Could you check a few things on this model? Use its own coordinates, in mm. Give positions to 0.01 mm unless a question says otherwise; leave off trailing zeros. Order: outer loops, then holes, each group sorted by start corner. A loop starts at its lowest first (then second) coordinate and runs counter-clockwise, first axis right, second up.
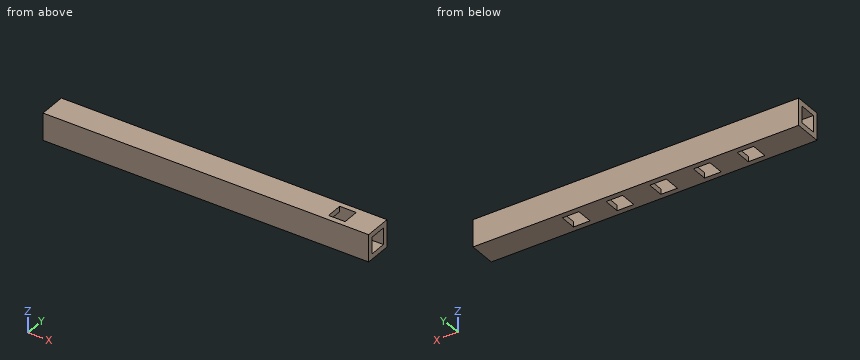
from build123d import *

# Parameters (mm, degrees)
F0_W      = 25.4
F0_H      = 25.4
F1_DEPTH  = 152.4
F1_FACE_W = 25.4
F1_FACE_H = 25.4
F2_DEPTH  = 152.4
F3_W      = 15.494
F3_H      = 15.494
F4_DEPTH  = 304.801
F5_W      = 15.494
F5_H      = 15.494
F6_DEPTH  = 19.05
F7_W      = 15.494
F7_H      = 15.494
F8_DEPTH  = 17.78
F9_DEPTH  = 15.24
F10_DEPTH = 15.24
F11_DEPTH = 15.24
F13_DEPTH = 15.24


with BuildPart() as f1:
    # F0 (on Right) → F1 (new body)
    with BuildSketch(Plane.YZ):
        with Locations((-3.156137, 12.7)):
            Rectangle(F0_W, F0_H)
    extrude(amount=-F1_DEPTH)

    # F1_face (on face) → F2 (join)
    with BuildSketch(Plane(origin=(0, -3.156137, 12.7), x_dir=(0, 1, 0), z_dir=(1, 0, 0))):
        Rectangle(F1_FACE_W, F1_FACE_H)
    extrude(amount=F2_DEPTH)

    # F3 (on face) → F4 (cut, through all)
    with BuildSketch(Plane.YZ.offset(152.4)):
        with Locations((-3.156137, 12.7)):
            Rectangle(F3_W, F3_H)
    extrude(amount=-F4_DEPTH, mode=Mode.SUBTRACT)

    # F5 (on face) → F6 (cut)
    with BuildSketch(Plane(origin=(0, 0, 0), x_dir=(1, 0, 0), z_dir=(0, 0, -1))):
        with Locations((-99.187, 3.156137)):
            Rectangle(F5_W, F5_H)
    extrude(amount=-F6_DEPTH, mode=Mode.SUBTRACT)

    # F7 (on face) → F8 (cut)
    with BuildSketch(Plane(origin=(0, 0, 0), x_dir=(1, 0, 0), z_dir=(0, 0, -1))):
        with Locations((-58.293, 3.156137)):
            Rectangle(F7_W, F7_H)
    extrude(amount=-F8_DEPTH, mode=Mode.SUBTRACT)

    # F7 (on face) → F9 (cut)
    with BuildSketch(Plane(origin=(0, 0, 0), x_dir=(1, 0, 0), z_dir=(0, 0, -1))):
        with Locations((-17.399, 3.156137)):
            Rectangle(F7_W, F7_H)
    extrude(amount=-F9_DEPTH, mode=Mode.SUBTRACT)

    # F7 (on face) → F10 (cut)
    with BuildSketch(Plane(origin=(0, 0, 0), x_dir=(1, 0, 0), z_dir=(0, 0, -1))):
        with Locations((23.495, 3.156137)):
            Rectangle(F7_W, F7_H)
    extrude(amount=-F10_DEPTH, mode=Mode.SUBTRACT)

    # F7 (on face) → F11 (cut)
    with BuildSketch(Plane(origin=(0, 0, 0), x_dir=(1, 0, 0), z_dir=(0, 0, -1))):
        with Locations((64.389, 3.156137)):
            Rectangle(F7_W, F7_H)
    extrude(amount=-F11_DEPTH, mode=Mode.SUBTRACT)

    # F12 (on face) → F13 (cut)
    with BuildSketch(Plane.XY.offset(25.4)):
        Polygon((127, -10.903137), (127, -3.156137), (127, 4.590863), (111.506, 4.590863), (111.506, -10.903137), align=None)
    extrude(amount=-F13_DEPTH, mode=Mode.SUBTRACT)


solid = f1.part
Item 1: For pin 1 (6 mm diameter, centred on y = -5.5, z = 17, fed in from -X); pin 2 (10 mm diameter, centred on x = -94, y = -2, fed in from -Z), each with a flat end and sliding along its axis, tell me the tip position at first contact or that it passes through.
Findings:
pin 1: passes through
pin 2: stops at z = 0
Item 2: Imagine slicing it at C-C on y = 0. Give the number of separate pieces and of enclosed holes in the cut face, then the cut area to 3 significant figures.
Findings:
separate pieces: 8
enclosed holes: 0
area: 2,560 mm2
Item 3: Imagine slicing it at A-A on x = 53. List the corners of the cut face in (y, z) for me.
Findings:
outline: (-15.86, 0) - (9.54, 0) - (9.54, 25.4) - (-15.86, 25.4) - close; hole (-10.9, 4.95) - (4.59, 4.95) - (4.59, 20.45) - (-10.9, 20.45) - close
Item 4: Please list where these lines run through material, in increasing order: line 1 along X through (y, z) = (3.5, 4.5); line 2 along Y through (x, z) = (26.5, 16.5); line 3 along X through (y, z) = (0.25, 21.5).
Findings:
line 1: x = -152.4 to -106.93, -91.44 to -66.04, -50.55 to -25.15, -9.65 to 15.75, 31.24 to 56.64, 72.14 to 152.4
line 2: y = -15.86 to -10.9, 4.59 to 9.54
line 3: x = -152.4 to 111.51, 127 to 152.4
Item 5: Imagine slicing it at B-B on z = 16.25. List the corners of the cut face in (x, y) for me, then the cut area to 3 significant figures.
Findings:
outline: (-152.4, -15.86) - (152.4, -15.86) - (152.4, -10.9) - (-152.4, -10.9) - close; (-152.4, 4.59) - (152.4, 4.59) - (152.4, 9.54) - (-152.4, 9.54) - close
area: 3,020 mm2
Item 6: Imagine slicing it at D-D on x = -99.5. List the corners of the cut face in (y, z) for me.
Findings:
outline: (-15.86, 0) - (-10.9, 0) - (-10.9, 20.45) - (4.59, 20.45) - (4.59, 0) - (9.54, 0) - (9.54, 25.4) - (-15.86, 25.4) - close
